Read the model definition and answer for the solid it produces. Units are mm, in the model's axes. Give positions to 0.01 mm unless a question says otherwise; leave off trailing zeros. Loops run counter-clockwise (first coordinate to the right, second up) from the corner with the lowest first, then second, coordinate; pieces in that order, holes last. Notation, with made-up numbers: (-40, 18) - (2, 18) arc R24 cw to (2, 40) - close; hole circle Ø5 at (51, 14.25). An arc over 180 degrees is marked (long way). Write item = value, one per line.
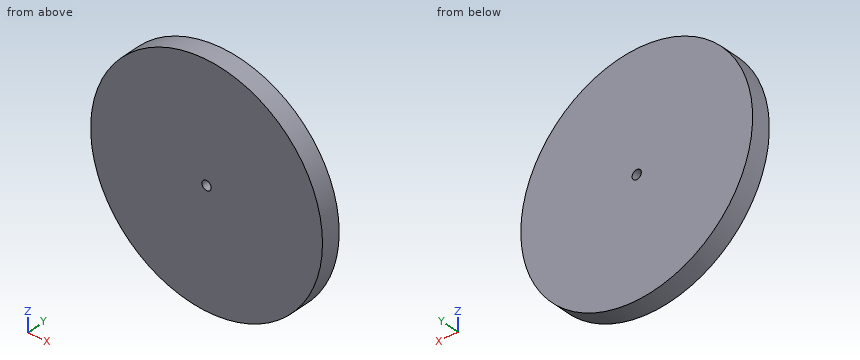
```python
from build123d import *

# Parameters (mm, degrees)
F0_R     = 60.459431
F2_DEPTH = 5
F1_R     = 2.4
F3_DEPTH = 5
F4_DEPTH = 25
F5_DEPTH = 25


with BuildPart() as f2:
    # F0 (on Front) → F2 (new body, symmetric)
    with BuildSketch(Plane.XZ):
        Circle(F0_R)
    extrude(amount=F2_DEPTH, both=True)

    # F1 (on face) → F3 (join, through all)
    with BuildSketch(Plane.XZ):
        Circle(F1_R)
    extrude(amount=F3_DEPTH)

    # F1 (on face) → F4 (cut)
    with BuildSketch(Plane.XZ):
        Circle(F1_R)
    extrude(amount=-F4_DEPTH, mode=Mode.SUBTRACT)

    # F1 (on face) → F5 (cut)
    with BuildSketch(Plane.XZ):
        Circle(F1_R)
    extrude(amount=F5_DEPTH, mode=Mode.SUBTRACT)


solid = f2.part
```
1) A cutting plane is placed at A-A on z = 0. Determine the outline of the cut face in (x, y), then the cut area to 3 significant figures.
Output:
outline = (-60.46, -5) - (-2.4, -5) - (-2.4, 5) - (-60.46, 5) - close; (2.4, -5) - (60.46, -5) - (60.46, 5) - (2.4, 5) - close
area = 1,160 mm²
2) Each of these flat-tipped pins is pushed along its axis until it touches: P1, Ø5, axis at x = 20.5, y = -3.5, coming from the +Z side; P2, Ø5, axis at y = 1.5, z = 18, coming from the -X side; P3, Ø1.5, axis at x = -38.5, y = -1.5, coming from the +Z side; P4, Ø7.5, axis at x = 0, z = 0, coming from the +Y side. Where does it stop, or does it pass through?
Output:
P1 = 57.72
P2 = -58.44
P3 = 47.23
P4 = 5
3) A cutting plane is placed at C-C on y = -3.5. Determine the outline of the cut face in (x, z), then the cut area to 3 significant figures.
Output:
outline = circle Ø120.92 at (0, 0); hole circle Ø4.8 at (0, 0)
area = 11,500 mm²
4) A cutting plane is placed at B-B on x = 0. Determine the outline of the cut face in (y, z), then the cut area to 3 significant figures.
Output:
outline = (-5, -60.46) - (5, -60.46) - (5, -2.4) - (-5, -2.4) - close; (-5, 2.4) - (5, 2.4) - (5, 60.46) - (-5, 60.46) - close
area = 1,160 mm²
5) A cutting plane is placed at D-D on z = 30.5. Determine the outline of the cut face in (x, y).
Output:
outline = (-52.2, -5) - (52.2, -5) - (52.2, 5) - (-52.2, 5) - close
6) Find the intervals of material crossed by probe 1 along Z at (x, y) = (0, 0.5); probe 2 along X at (y, z) = (1, 40); probe 3 along Z at (x, y) = (18, -1.75), in increasing order.
Output:
probe_1 = -60.46 to -2.4, 2.4 to 60.46
probe_2 = -45.34 to 45.34
probe_3 = -57.72 to 57.72
